Can you work these out from the model? Positions are in its coordinate system, mm. Face numbers are marked on the shaded views. Round coordinates to 2 decimals unless told otherwise and drop trailing zeros. Loops run counter-clockwise (first coordinate to the right, second up) from the corner with the lowest first, then second, coordinate; pieces in that order, holes last. Notation, with made-up numbers: M 74,22.5 L 108,22.5 A21 cw 108,33.5 Z; hole C 69,26.5 d2. An arc over 180 degrees is marked long. Return JSON: item names as keys, results as strings.
Autodesk Inventor part; units mm, degrees
ref_plane "YZ Plane" through (0, 0, 0) normal (1, 0, 0) x (0, 1, 0)
ref_plane "XZ Plane" through (0, 0, 0) normal (0, 1, 0) x (-1, 0, 0)
ref_plane "XY Plane" through (0, 0, 0) normal (0, 0, 1) x (1, 0, 0)
sketch "Sketch1" plane through (0, 0, 0) normal (0, 0, 1) x (1, 0, 0)
  line L0 (0, 0) -> (-63.5, 0)
  line L1 (-63.5, 0) -> (-63.5, 15.875)
  line L2 (-63.5, 15.875) -> (0, 15.875)
  line L3 (0, 15.875) -> (0, 0)
  line L4 (0, 6.2865) -> (-63.5, 6.2865)
  line L5 (-63.5, 6.2865) -> (-63.5, 9.5885)
  line L6 (-63.5, 9.5885) -> (0, 9.5885)
  line L7 (0, 9.5885) -> (0, 6.2865)
  line L8 (-47.625, 15.875) -> (-15.875, 15.875)
  line L9 (-15.875, 15.875) -> (-15.875, 0)
  line L10 (-15.875, 0) -> (-47.625, 0)
  line L11 (-47.625, 0) -> (-47.625, 15.875)
  circle A0 centre (-31.75, 7.9375) radius 6.35
  circle A1 centre (-31.75, 7.9375) radius 2.5797
  line L12 (-6.35, 6.2865) -> (-6.35, 9.5885)
  line L13 (-57.15, 6.2865) -> (-57.15, 9.5885)
  point P0 (-15.875, 6.2865)
  point P1 (-15.875, 9.5885)
  point P2 (-47.625, 9.5885)
  point P3 (-47.625, 6.2865)
  dimension "d12" = 15.875
  dimension "d13" = 6.2865
  dimension "d14" = 3.302
  dimension "d15" = 15.875
  dimension "d16" = 15.875
  dimension "d17" = 7.9375
  dimension "d18" = 31.75
  dimension "d19" = 12.7
  dimension "d20" = 5.1594
  dimension "d33" = 6.35
  dimension "d34" = 6.35
  dimension "d35" = 50.8
  dimension "d36" = 63.5
extrude "Extrusion1" add sketch "Sketch1" along normal blind 9.525 contours L0 L9 L4 L3 | L0 L11 L4 A0 L9 | L0 L1 L4 L11 | L4 A0 L6 L9 | L6 L9 L2 L3 | L11 L6 A0 L4 | A0 L4 A1 | L4 A1 L6 A0 | L6 A0 L11 L2 L9 | A0 L6 A1 L4 | L6 L1 L2 L11 | L6 A1 A0
sketch "Sketch2" plane through (-63.5, 15.875, 0) normal (0, 1, 0) x (1, 0, 0)
  circle A0 centre (57.15, -4.7625) radius 2.5797
  circle A1 centre (6.35, -4.7625) radius 2.5797
  line L0 (63.5, 0) -> (0, 0)
  line L1 (63.5, 0) -> (63.5, -9.525)
  line L2 (0, 0) -> (0, -9.525)
  dimension "d25" = 4.7625
  dimension "d26" = 4.7625
  dimension "d27" = 6.35
  dimension "d28" = 6.35
  dimension "d29" = 5.1594
extrude "Extrusion3" cut sketch "Sketch2" against normal through all
fillet "Fillet2" radius 1.5875 8 edges at (-63.5, 0, 4.7625) (-63.5, 6.2865, 4.7625) (-63.5, 9.5885, 4.7625) (-63.5, 15.875, 4.7625) (0, 15.875, 4.7625) (0, 9.5885, 4.7625) (0, 6.2865, 4.7625) (0, 0, 4.7625)
equation "\"d13\" = -0.5 * d14 + 0.5 * d12"
equation "\"d16\" = d15"
equation "\"d17\" = 0.5 * d12"
equation "\"d18\" = 0.5 * d36"
equation "\"d33\" = d34"
equation "\"d26\" = d25"
equation "\"d27\" = d28"
properties part number "Connector"
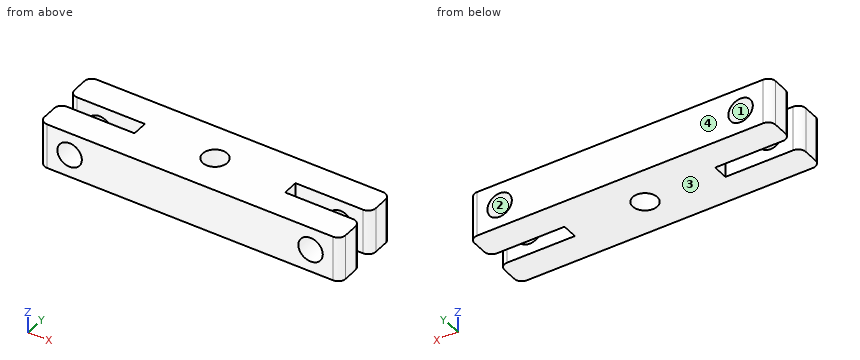
Q1. I'm going to push flat-ended pins straight in: pin 1 Ø4.5 at (x, z) = (-57.15, 4.76) entering from +Y; pin 2 Ø1.7 at (y, z) = (8.5, 4.5) entering from -X (3 decimals). Where does each tip first touch, or does it pass through?
Results:
{"pin 1": "passes through", "pin 2": "stops at x = -47.625"}
Q2. Suppose I cut it at A-A, the plane x = -6.35. Please give me the cut outline in (y, z) (1 decimal).
Results:
{"outline": "M 0,0 L 6.3,0 L 6.3,2.2 L 0,2.2 Z; M 0,7.3 L 6.3,7.3 L 6.3,9.5 L 0,9.5 Z; M 9.6,0 L 15.9,0 L 15.9,2.2 L 9.6,2.2 Z; M 9.6,7.3 L 15.9,7.3 L 15.9,9.5 L 9.6,9.5 Z"}
Q3. Suppose I cut it at B-B, the plane x = -31.75. Please give me the cut outline in (y, z) (3 decimals).
Results:
{"outline": "M 0,0 L 5.358,0 L 5.358,9.525 L 0,9.525 Z; M 10.517,0 L 15.875,0 L 15.875,9.525 L 10.517,9.525 Z"}
Q4. Suppose I cut it at D-D, the plane y = 2.5. State how many separate pieces and enclosed holes the cut face has, plus the area to 3 significant figures.
Results:
{"separate pieces": "1", "enclosed holes": "2", "area": "563 mm2"}
Q5. If I drill on line 1 along Y through (x, z) = (-13.5, 2) (1 decimal); line 2 along Z through (x, y) = (-6.35, 13.25) (3 decimals); line 3 along X through (y, z) = (5.25, 5.5), over which ranges is the centre line in solid material (lowest first)?
Results:
{"line 1": "y = 0 to 6.3, 9.6 to 15.9", "line 2": "z = 0 to 2.183, 7.342 to 9.525", "line 3": "x = -63.4 to -59.62, -54.68 to -8.82, -3.88 to -0.1"}
Q6. Thinking about a two-plate mould opening in Z: for the marked faces 1, 2, 3 and 4, which applies, pulls with the +Z half, pulls with the -Z half, needs draft (parallel to the pull), parting line crosses it, or undercut?
Results:
{"face 1": "undercut", "face 2": "undercut", "face 3": "pulls with the -Z half", "face 4": "needs draft"}
